Design review of the part built by this model. Coordinates are the model's own, in mm. A direction names the side the tool comes from. Give positions to 0.01 mm unless a question says otherwise; leave off trailing zeros. Loops run counter-clockwise (first coordinate to the right, second up) from the corner with the lowest first, then second, coordinate; pieces in that order, holes last.
from build123d import *

# Parameters (mm, degrees)
SKETCH_2_W                = 30
SKETCH_2_H                = 30
EXTRUDE_1_DEPTH           = 225
SKETCH_4_W                = 26
SKETCH_4_H                = 26
CUT_EXTRUDE_1_DEPTH       = 226
CUT_EXTRUDE_1_DEPTH_BACK  = 226
SKETCH_5_R                = 2.025
CUT_EXTRUDE_2_DEPTH       = 1
CUT_EXTRUDE_2_DEPTH_BACK  = 31
CUT_EXTRUDE_3_DEPTH       = 10
CUT_EXTRUDE_START         = -31
SKETCH_8_R                = 1.525
CUT_EXTRUDE_4_DEPTH       = 32
PATTERN_LINEAR_2_COUNT    = 13
PATTERN_LINEAR_2_PITCH    = 30
PATTERN_LINEAR_3_COUNT    = 7
PATTERN_LINEAR_3_PITCH    = 57
SKETCH_9_R                = 1.525
CUT_EXTRUDE_5_DEPTH       = 1
CUT_EXTRUDE_5_DEPTH_BACK  = 31
SKETCH_10_R               = 2.025
CUT_EXTRUDE_6_DEPTH       = 1
CUT_EXTRUDE_6_DEPTH_BACK  = 31
SKETCH_6_R                = 4
CUT_EXTRUDE_7_DEPTH       = 10
CUT_EXTRUDE_8_DEPTH       = 10
CUT_EXTRUDE_9_DEPTH       = 10
SKETCH_13_R               = 1.525
CUT_EXTRUDE_10_DEPTH      = 1
CUT_EXTRUDE_10_DEPTH_BACK = 31
SKETCH_14_R               = 7.5
CUT_EXTRUDE_11_DEPTH      = 2


with BuildPart() as part:
    # 草图2 → 凸台-拉伸1 (new body, symmetric)
    with BuildSketch(Plane(origin=(0, 0, 0), x_dir=(1, 0, 0), z_dir=(0, 1, 0))):
        Rectangle(SKETCH_2_W, SKETCH_2_H)
    extrude(amount=EXTRUDE_1_DEPTH, both=True)

    # 草图4 → 切除-拉伸1 (cut, two sides)
    with BuildSketch(Plane(origin=(0, 0, 0), x_dir=(1, 0, 0), z_dir=(0, 1, 0))) as cut_extrude_1_sk:
        Rectangle(SKETCH_4_W, SKETCH_4_H)
    extrude(amount=CUT_EXTRUDE_1_DEPTH, mode=Mode.SUBTRACT)
    extrude(cut_extrude_1_sk.sketch, amount=-CUT_EXTRUDE_1_DEPTH_BACK, mode=Mode.SUBTRACT)

    # 草图5 → 切除-拉伸2 (cut, two sides)
    with BuildSketch(Plane(origin=(0, 0, -15), x_dir=(-1, 0, 0), z_dir=(0, 0, -1))) as cut_extrude_2_sk:
        with Locations((-7.5, 210)):
            Circle(SKETCH_5_R)
        with Locations((7.5, 210)):
            Circle(SKETCH_5_R)
        with Locations((-7.5, 195)):
            Circle(SKETCH_5_R)
        with Locations((7.5, 195)):
            Circle(SKETCH_5_R)
    extrude(amount=CUT_EXTRUDE_2_DEPTH, mode=Mode.SUBTRACT)
    extrude(cut_extrude_2_sk.sketch, amount=-CUT_EXTRUDE_2_DEPTH_BACK, mode=Mode.SUBTRACT)

    # 草图7 → 切除-拉伸3 (cut)
    with BuildSketch(Plane(origin=(0, 0, -15), x_dir=(-1, 0, 0), z_dir=(0, 0, -1))):
        with BuildLine():
            Line((-9, -196.5), (-9, -165.5))
            ThreePointArc((-9, -165.5), (0, -156.5), (9, -165.5))
            Line((9, -165.5), (9, -196.5))
            ThreePointArc((9, -196.5), (0, -205.5), (-9, -196.5))
        make_face()
    cut_extrude_3 = extrude(amount=-CUT_EXTRUDE_3_DEPTH, mode=Mode.SUBTRACT)

    # 草图8 → 切除-拉伸4 (cut)
    with BuildSketch(Plane(origin=(15, 0, 0), x_dir=(0, 0, -1), z_dir=(1, 0, 0)).offset(CUT_EXTRUDE_START)):
        with Locations((0, -170.000000001)):
            Circle(SKETCH_8_R)
    cut_extrude_4 = extrude(amount=CUT_EXTRUDE_4_DEPTH, mode=Mode.SUBTRACT)

    # 阵列(线性)2: 切除-拉伸4 ×13
    with Locations(*[(0, i * PATTERN_LINEAR_2_PITCH, 0) for i in range(1, PATTERN_LINEAR_2_COUNT)]):
        add(cut_extrude_4, mode=Mode.SUBTRACT)

    # 阵列(线性)3: 切除-拉伸3 ×7
    with Locations(*[(0, i * PATTERN_LINEAR_3_PITCH, 0) for i in range(1, PATTERN_LINEAR_3_COUNT)]):
        add(cut_extrude_3, mode=Mode.SUBTRACT)

    # 草图9 → 切除-拉伸5 (cut, two sides)
    with BuildSketch(Plane(origin=(15, 0, 0), x_dir=(0, 0, -1), z_dir=(1, 0, 0))) as cut_extrude_5_sk:
        with Locations((6.5, 202.5)):
            Circle(SKETCH_9_R)
        with Locations((-6.5, 202.5)):
            Circle(SKETCH_9_R)
    extrude(amount=CUT_EXTRUDE_5_DEPTH, mode=Mode.SUBTRACT)
    extrude(cut_extrude_5_sk.sketch, amount=-CUT_EXTRUDE_5_DEPTH_BACK, mode=Mode.SUBTRACT)

    # 草图10 → 切除-拉伸6 (cut, two sides)
    with BuildSketch(Plane(origin=(15, 0, 0), x_dir=(0, 0, -1), z_dir=(1, 0, 0))) as cut_extrude_6_sk:
        with Locations((9, -187)):
            Circle(SKETCH_10_R)
        with Locations((-9, -187)):
            Circle(SKETCH_10_R)
        with Locations((-9, -217)):
            Circle(SKETCH_10_R)
        with Locations((9, -217)):
            Circle(SKETCH_10_R)
    extrude(amount=CUT_EXTRUDE_6_DEPTH, mode=Mode.SUBTRACT)
    extrude(cut_extrude_6_sk.sketch, amount=-CUT_EXTRUDE_6_DEPTH_BACK, mode=Mode.SUBTRACT)

    # 草图6 → 切除-拉伸7 (cut)
    with BuildSketch(Plane(origin=(0, 0, -15), x_dir=(-1, 0, 0), z_dir=(0, 0, -1))):
        with Locations((-7.5, 210)):
            Circle(SKETCH_6_R)
        with Locations((-7.5, 195)):
            Circle(SKETCH_6_R)
        with Locations((7.5, 195)):
            Circle(SKETCH_6_R)
        with Locations((7.5, 210)):
            Circle(SKETCH_6_R)
    extrude(amount=-CUT_EXTRUDE_7_DEPTH, mode=Mode.SUBTRACT)

    # 草图11 → 切除-拉伸8 (cut)
    with BuildSketch(Plane.XY.offset(15)):
        with BuildLine():
            Line((-9, 125), (-9, 135))
            ThreePointArc((-9, 135), (0, 144), (9, 135))
            Line((9, 135), (9, 125))
            ThreePointArc((9, 125), (0, 116), (-9, 125))
        make_face()
        with BuildLine():
            Line((-9, 65), (-9, 75))
            ThreePointArc((-9, 75), (0, 84), (9, 75))
            Line((9, 75), (9, 65))
            ThreePointArc((9, 65), (0, 56), (-9, 65))
        make_face()
        with BuildLine():
            Line((-9, 5), (-9, 15))
            ThreePointArc((-9, 15), (0, 24), (9, 15))
            Line((9, 15), (9, 5))
            ThreePointArc((9, 5), (0, -4), (-9, 5))
        make_face()
    extrude(amount=-CUT_EXTRUDE_8_DEPTH, mode=Mode.SUBTRACT)

    # 草图12 → 切除-拉伸9 (cut)
    with BuildSketch(Plane.XY.offset(15)):
        with BuildLine():
            Line((-6, 170), (6, 170))
            ThreePointArc((6, 170), (8.121320344, 170.878679656), (9, 173))
            Line((9, 173), (9, 187))
            ThreePointArc((9, 187), (8.121320344, 189.121320344), (6, 190))
            Line((6, 190), (-6, 190))
            ThreePointArc((-6, 190), (-8.121320344, 189.121320344), (-9, 187))
            Line((-9, 187), (-9, 173))
            ThreePointArc((-9, 173), (-8.121320344, 170.878679656), (-6, 170))
        make_face()
    extrude(amount=-CUT_EXTRUDE_9_DEPTH, mode=Mode.SUBTRACT)

    # 草图13 → 切除-拉伸10 (cut, two sides)
    with BuildSketch(Plane(origin=(0, 0, -15), x_dir=(-1, 0, 0), z_dir=(0, 0, -1))) as cut_extrude_10_sk:
        with Locations((0.05, 202.5)):
            Circle(SKETCH_13_R)
    extrude(amount=CUT_EXTRUDE_10_DEPTH, mode=Mode.SUBTRACT)
    extrude(cut_extrude_10_sk.sketch, amount=-CUT_EXTRUDE_10_DEPTH_BACK, mode=Mode.SUBTRACT)

    # 草图14 → 切除-拉伸11 (cut)
    with BuildSketch(Plane(origin=(0, 0, 13), x_dir=(-1, 0, 0), z_dir=(0, 0, -1))):
        with Locations((0, -200)):
            Circle(SKETCH_14_R)
    extrude(amount=-CUT_EXTRUDE_11_DEPTH, mode=Mode.SUBTRACT)


solid = part.part
Q1. Draft analysis for pull direction Y (two halves, no side actions). For faces 1 (the face through (-14, -225, 0)), 2 (the face through (0.198, -42.502, -14.014)), 3 (the face through (13, 3, 0)), state which applies: pulls with the +Y half, pulls with the -Y half, needs draft (parallel to the pull), parting line crosses it, or undercut.
Results:
face 1: pulls with the -Y half
face 2: undercut
face 3: needs draft
Q2. Tool access review of faces 4 (the face through (-9, 3, 13)), 5 (the face through (-6.979, 213.966, -14.014)), 6 (the face through (0, 84, 14)): name each direction out of +Z, -Z, +X, -X, +Y, -Y from which nothing blocks a thin tool from reaching the whole face with its end or side.
Results:
face 4: +Y, -Y
face 5: -Z
face 6: +Z
Q3. Insertion check: pin 1 (1 mm diameter, centred on x = -5.5, y = 161, fed in from -Z). The pin has a flat end and moves straight along its axis. Give the tip position at first contact, or say it passes through.
Results:
pin 1: stops at z = 13
Q4. Take a section at A-A (y = -62.5). Give the boundary of the cut face in (x, z), plus the area to 3 significant figures.
Results:
outline: (-15, -15) - (-9, -15) - (-9, -13) - (-13, -13) - (-13, 13) - (13, 13) - (13, -13) - (9, -13) - (9, -15) - (15, -15) - (15, 15) - (-15, 15) - close
area: 188 mm2
Q5. Wall thickness on line 1 (Z direction, x = 14.3, y = 202.5) (3 decimals); line 2 (Z direction, x = 14.25, y = -217) (3 decimals); line 3 (X direction, y = 21.5, z = -3.25): over which ranges is each line inside the solid? List them lowest first.
Results:
line 1: z = -15 to -8.025, -4.975 to 4.975, 8.025 to 15
line 2: z = -15 to -11.025, -6.975 to 6.975, 11.025 to 15
line 3: x = -15 to -13, 13 to 15
